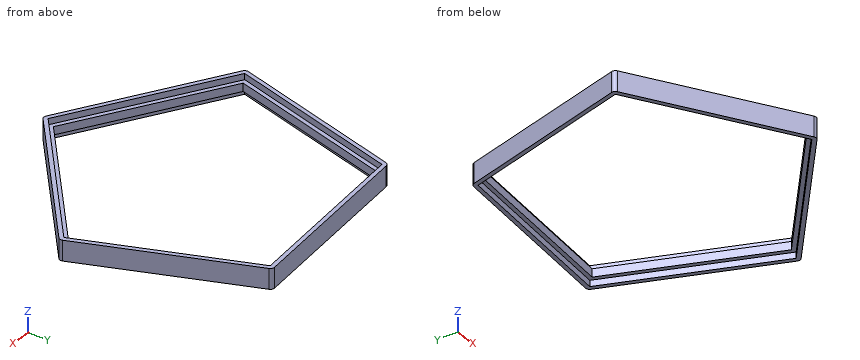
from build123d import *

# Parameters (mm, degrees)
F1_DEPTH = 1
F2_DEPTH = 2.5
F3_R     = 1


with BuildPart() as f1:
    # F0 (on Top) → F1 (new body, symmetric)
    with BuildSketch(Plane.XY):
        Polygon((19.571643256, 31.4964826728), (-23.9069647124, 28.3466872622), (-34.3469600161, -13.9772664763), (2.6793760122, -36.9851130144), (36.0029054603, -8.8807904443), align=None)
        Polygon((-33.2106868902, -13.4901422574), (-23.0925543436, 27.4165569635), (18.9387034188, 30.4345063154), (34.7973167593, -8.6069976298), (2.5672210558, -35.7539233917), align=None, mode=Mode.SUBTRACT)
        Polygon((18.9387034188, 30.4345063154), (-23.0925543436, 27.4165569635), (-33.2106868902, -13.4901422574), (2.5672210558, -35.7539233917), (34.7973167593, -8.6069976298), align=None)
        Polygon((-32.949379101, -13.3121576596), (-22.8425323844, 27.2230387533), (18.8319176983, 30.1369208862), (34.4812975953, -8.5973973294), (2.4786961918, -35.4504046505), align=None, mode=Mode.SUBTRACT)
        Polygon((18.8319176983, 30.1369208862), (-22.8425323844, 27.2230387533), (-32.949379101, -13.3121576596), (2.4786961918, -35.4504046505), (34.4812975953, -8.5973973294), align=None)
        Polygon((-32.0654907905, -13.0249649382), (-22.2962593663, 26.4711584475), (18.2856446802, 29.3850405804), (33.5974092848, -8.310204608), (2.4786961918, -34.5210294816), align=None, mode=Mode.SUBTRACT)
    extrude(amount=F1_DEPTH, both=True)

    # F0 (on Top) → F2 (join, symmetric)
    with BuildSketch(Plane.XY):
        Polygon((19.571643256, 31.4964826728), (-23.9069647124, 28.3466872622), (-34.3469600161, -13.9772664763), (2.6793760122, -36.9851130144), (36.0029054603, -8.8807904443), align=None)
        Polygon((-33.2106868902, -13.4901422574), (-23.0925543436, 27.4165569635), (18.9387034188, 30.4345063154), (34.7973167593, -8.6069976298), (2.5672210558, -35.7539233917), align=None, mode=Mode.SUBTRACT)
    extrude(amount=F2_DEPTH, both=True)

    # F3
    f3_edges = [f1.edges().sort_by_distance(p)[0] for p in [
        (36.002905, -8.88079, 0),
        (2.679376, -36.985113, 0),
        (-34.34696, -13.977266, 0),
        (-23.906965, 28.346687, 0),
        (19.571643, 31.496483, 0),
    ]]
    fillet(f3_edges, radius=F3_R)


solid = f1.part
The listing builds one solid part. Answer for the finished solid, in the listing's coordinates (mm). Give positions to 0.01 mm unless a question says otherwise; leave off trailing zeros. Order: outer loops, then holes, each group sorted by start corner. A loop starts at its lowest first (then second) coordinate and runs counter-clockwise, first axis right, second up. Notation, with made-up numbers: (75.5, -9.5) - (88.5, -9.5) arc R36 cw to (88.5, 25.5) - close; hole circle Ø8 at (34, 33). An arc over 180 degrees is marked (long way). One line per item, written item: value. Start each with the question number.
1) Find the intervals of material crossed by L1, parallel to X at y = 16, z = -1.35; L2, parallel to X at y = 12, z = 1.6; L3, parallel to Y at x = -11.5, z = 0, in increasing order.
2) A cutting plane is placed at B-B on y = -25. Give the vertices of the cut face in (x, z), then the cut area to 3 significant figures.
3) A cutting plane is placed at A-A on x = -5. Give the vertices of the cut face in (y, z), then the cut area to 3 significant figures.
4) Given pin 1 Ø2 at (y, z) = (10, 0.5) entering from +X; pin 2 Ø3 at (x, y) = (-6.5, -28) entering from +Z, each flat-ended and moving along its own axis, determine where each tip first touches the part or whether it passes through.
Answer sheet:
1. L1: x = -26.95 to -25.92, 24.8 to 25.88
1. L2: x = -27.94 to -26.91, 26.43 to 27.51
1. L3: y = -28.17 to -25.82, 27.25 to 29.25
2. outline: (-16.61, -2.5) - (-14.71, -2.5) - (-14.71, -1) - (-12.82, -1) - (-12.82, 1) - (-14.71, 1) - (-14.71, 2.5) - (-16.61, 2.5) - close; (13.78, -1) - (15.33, -1) - (15.33, -2.5) - (16.89, -2.5) - (16.89, 2.5) - (15.33, 2.5) - (15.33, 1) - (13.78, 1) - close
2. area: 24.1 mm2
3. outline: (-32.21, -2.5) - (-31.05, -2.5) - (-31.05, -1) - (-29.87, -1) - (-29.87, 1) - (-31.05, 1) - (-31.05, 2.5) - (-32.21, 2.5) - close; (27.71, -1) - (28.72, -1) - (28.72, -2.5) - (29.72, -2.5) - (29.72, 2.5) - (28.72, 2.5) - (28.72, 1) - (27.71, 1) - close
3. area: 15.2 mm2
4. pin 1: stops at x = 28.73
4. pin 2: stops at z = 1
